Input: part model. Units: mm. Frame: model coordinates. Face numbers are marked on the shaded views. A direction names the side the tool comes from. Coordinates: 2 decimals unless noted, no trailing zeros. Loops run counter-clockwise (first coordinate to the right, second up) from the corner with the lowest first, then second, coordinate; pieces in that order, holes last.
```python
from build123d import *

# Parameters (mm, degrees)
SKETCH1_R           = 2.5
BOSS_EXTRUDE1_DEPTH = 5
SKETCH2_R           = 2.5
BOSS_EXTRUDE2_DEPTH = 5


with BuildPart() as part:
    # Sketch1 → Boss-Extrude1 (new body)
    with BuildSketch(Plane(origin=(0, 0, 0), x_dir=(1, 0, 0), z_dir=(0, 1, 0))):
        with BuildLine():
            Line((-14.504443595, 6.706697569), (27.895556405, 6.137023864))
            ThreePointArc((27.895556405, 6.137023864), (32.82793273, 1.070302658), (27.761211524, -3.862073668))
            Line((27.761211524, -3.862073668), (-14.638788476, -3.292399963))
            ThreePointArc((-14.638788476, -3.292399963), (-19.571164802, 1.774321243), (-14.504443595, 6.706697569))
        make_face()
        with Locations(Location((-14.571616036, 1.707148803, 0), (0, 0, 270))):
            Circle(SKETCH1_R, mode=Mode.SUBTRACT)
    extrude(amount=BOSS_EXTRUDE1_DEPTH)

    # Sketch2 → Boss-Extrude2 (add)
    with BuildSketch(Plane(origin=(0, 5, 0), x_dir=(1, 0, 0), z_dir=(0, 1, 0))):
        with Locations(Location((27.828383964, 1.137475098, 0), (0, 0, 270))):
            Circle(SKETCH2_R)
    extrude(amount=BOSS_EXTRUDE2_DEPTH)


solid = part.part
```
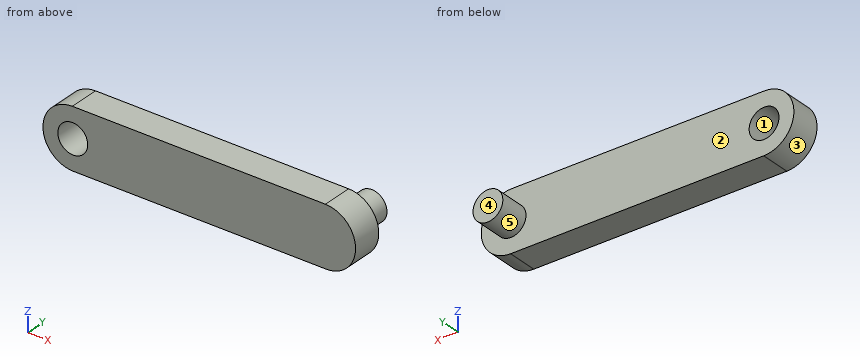
Item 1: Section query A-A (x = -16). Output: boundary loops of the cut face in (y, z).
Result:
outline: (0, -6.5) - (5, -6.5) - (5, -3.76) - (0, -3.76) - close; (0, 0.34) - (5, 0.34) - (5, 3.08) - (0, 3.08) - close
Item 2: Section query C-C (z = -5). Output: boundary loops of the cut face in (x, y).
Result:
outline: (-18.33, 0) - (31, 0) - (31, 5) - (-18.33, 5) - close
Item 3: Section query D-D (y = 8.5). Output: boundary loops of the cut face in (x, z), then the cut area to 3 significant figures.
Result:
outline: circle Ø5 at (27.83, -1.14)
area: 19.6 mm2
Item 4: Section query B-B (y = 1.5). Output: boundary loops of the cut face in (x, z).
Result:
outline: (-14.64, 3.29) arc R5 ccw to (-14.5, -6.71) - (27.9, -6.14) arc R5 ccw to (27.76, 3.86) - close; hole circle Ø5 at (-14.57, -1.71)
Item 5: Contact query for flat-ended pins moving along their axis: P1, Ø5, axis at x = 21, y = 6.5, coming from the -Z side; P2, Ø5.5, axis at x = -2.5, z = -1.5, coming from the +Y side; P3, Ø1, axis at x = 23.5, y = 3, coming from the -Z side; P4, Ø4, axis at x = -13, y = 7.5, coming from the -Z side. Output: stop coordinate, or through.
Result:
P1: stops at z = -6.26
P2: stops at y = 5
P3: stops at z = -6.2
P4: passes through
Item 6: Line query: L1, parallel to Y at x = 28, z = 2.75; L2, parallel to X at y = 1, z = -0.75; L3, parallel to X at y = 1.75, z = -5.5. Output: solid intervals per line, ascending.
Result:
L1: y = 0 to 5
L2: x = -19.48 to -16.88, -12.26 to 32.81
L3: x = -17.83 to 30.27
Item 7: Reachability of the marked faces 4 and 5 from +Z, -Z, +X, -X, +Y, -Y: full face, straight path, thin tool, end or side. Return the list, or none.
Result:
face 4: +Z, -Z, +X, -X, +Y
face 5: +Y
Item 8: Mould query, pull axis Z, two halves, no side actions, for the marked faces 1, 2 and 3. Classes: +Z half, -Z half, draft (parallel to the pull), parting line (faces both ways), or undercut.
Result:
face 1: undercut
face 2: draft
face 3: parting line
